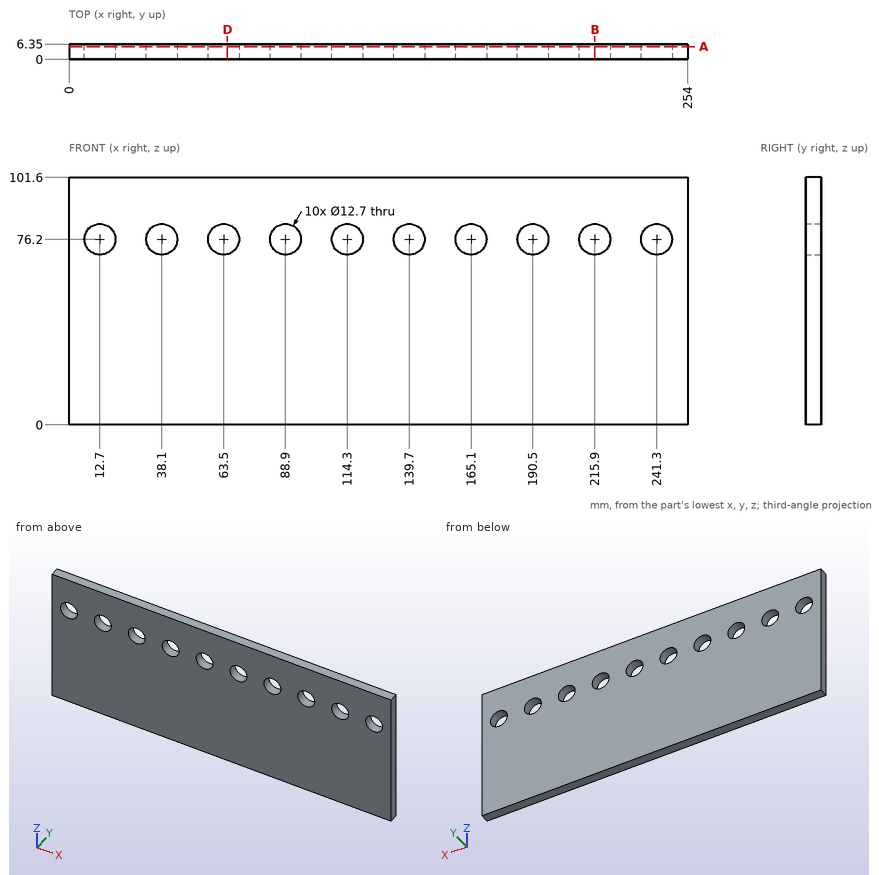
Input: dimensioned drawing with shaded views. Units: mm. Origin: part minimum x, y, z. Give positions to 0.01 mm unless a question says otherwise; leave off trailing zeros. Loops run counter-clockwise (first coordinate to the right, second up) from the corner with the lowest first, then second, coordinate; pieces in that order, holes last. Notation, with made-up numbers: M 11,65.25 L 35,65.25 A28 cw 35,97.25 Z; hole C 41,21 d10. An arc over 180 degrees is marked long. Put each result on its own line as item: value. Start each with the question number.
1) Cut plane D-D (x = 65). Output: boundary loops of the cut face in (y, z).
2) Cut plane B-B (x = 215.9). Output: boundary loops of the cut face in (y, z).
3) Cut plane A-A (y = 5.25). Give the number of separate pieces and of enclosed holes in the cut face, then the cut area to 3 significant figures.
4) Ray query, line 1 along Z through (x, y) = (38.5, 1.5); line 2 along Z through (x, y) = (65.5, 5.5). Return the intervals inside material, ascending.
Verdict:
1. outline: M 0,0 L 6.35,0 L 6.35,70.03 L 0,70.03 Z; M 0,82.37 L 6.35,82.37 L 6.35,101.6 L 0,101.6 Z
2. outline: M 0,0 L 6.35,0 L 6.35,69.85 L 0,69.85 Z; M 0,82.55 L 6.35,82.55 L 6.35,101.6 L 0,101.6 Z
3. separate pieces: 1
3. enclosed holes: 10
3. area: 24,500 mm2
4. line 1: 0 to 69.86, 82.54 to 101.6
4. line 2: 0 to 70.17, 82.23 to 101.6
